Here's the drawing with two shaded views (mm, measured from the low corner). I have some questions. Round coordinates to 2 decimals unless told otherwise and drop trailing zeros. Order: outer loops, then holes, each group sorted by start corner. A loop starts at its lowest first (then second) coordinate and runs counter-clockwise, first axis right, second up.
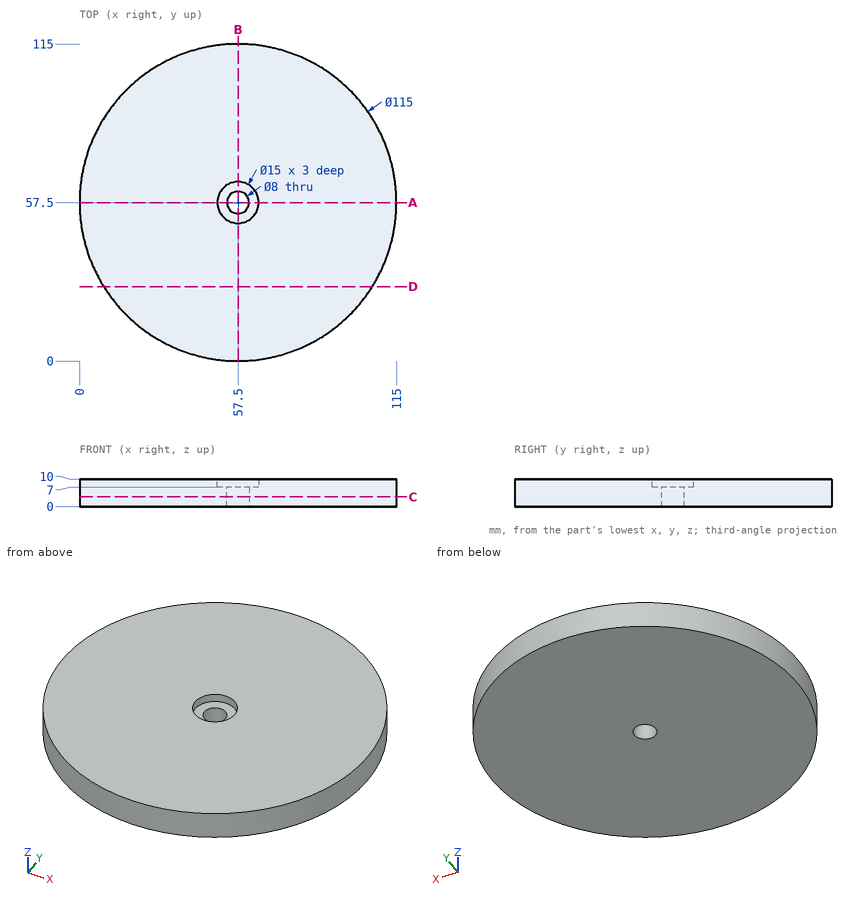
1. If we section it at A-A, the plane y = 57.5: Write out the boundary of the cut face in (x, z), and give its area (3 significant figures).
Evaluation:
outline: (0, 0) - (53.5, 0) - (53.5, 7) - (50, 7) - (50, 10) - (0, 10) - close; (61.5, 0) - (115, 0) - (115, 10) - (65, 10) - (65, 7) - (61.5, 7) - close
area: 1,050 mm2
2. If we section it at D-D, the plane y = 27: Write out the boundary of the cut face in (x, z), and give its area (3 significant figures).
Evaluation:
outline: (8.76, 0) - (106.24, 0) - (106.24, 10) - (8.76, 10) - close
area: 975 mm2
3. I'm going to push flat-ended pins straight in: P1, Ø4, axis at y = 14.5, z = 4.5, coming from the -X side; P2, Ø6, axis at y = 22, z = 3, coming from the +X side; P3, Ø4, axis at x = 95.5, z = 8.5, coming from the -Y side. Where does each tip first touch, or does it pass through?
Evaluation:
P1: stops at x = 17.19
P2: stops at x = 104.93
P3: stops at y = 12.66
4. If we section it at C-C, the plane z = 3.5: Write out the boundary of the cut face in (x, y), and give its area (3 significant figures).
Evaluation:
outline: circle Ø115 at (57.5, 57.5); hole circle Ø8 at (57.5, 57.5)
area: 10,300 mm2
5. I need wall thicknesses on probe 1 along Y at (x, z) = (57.5, 4.75); probe 2 along Y at (x, z) = (57.5, 8.5); probe 3 along X at (y, z) = (91, 8.5). Which ranges of each line are inside material? Lowest first, please.
Evaluation:
probe 1: y = 0 to 53.5, 61.5 to 115
probe 2: y = 0 to 50, 65 to 115
probe 3: x = 10.77 to 104.23
